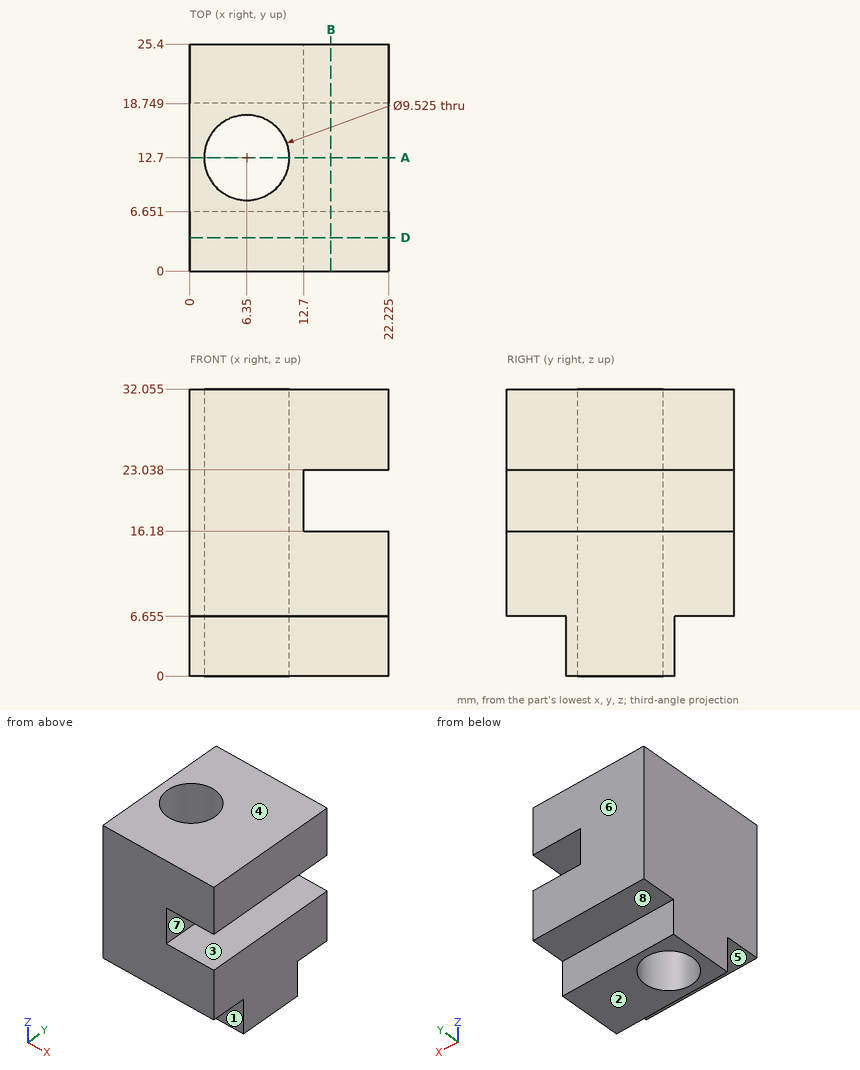
The figure shows three views and two pictorial views of one solid part (mm, origin at its lowest corner). Answer the questions. A direction names the side the tool comes from. Give positions to 0.01 mm unless a question says otherwise; leave off trailing zeros. Loops run counter-clockwise (first coordinate to the right, second up) from the corner with the lowest first, then second, coordinate; pieces in that order, holes last. Notation, with made-up numbers: (7, 34) -> (48, 34) arc R7 cw to (48, 47) -> close; hole circle Ø5 at (5.25, 51.5). An arc over 180 degrees is marked (long way). Put each result on its own line as item: value. Start each with the question number.
Item 1: Find the intervals of material crossed by L1, parallel to X at y = 12.7, z = 7 (1 decimal); L2, parallel to Z at x = 14.5, y = 13.75 (1 decimal); L3, parallel to Z at x = 19.5, y = 5.5 (1 decimal), in increasing order. Write a range as [from, to].
Item 2: Each of these flat-tipped pins is pushed along its axis until it touches: P1, Ø5.5, axis at x = 15, z = 2, coming from the +Y side; P2, Ø10, axis at y = 20, z = 13.5, coming from the -X side; P3, Ø3.5, axis at x = 10, y = 21, coming from the -Z side (3 decimals); P4, Ø2, axis at x = 5.5, z = 2, coming from the -Y side. Where does it stop, or does it pass through?
Item 3: Which of the six approach directions +Z, -Z, +X, -X, +Y, -Y give full straight-line access (tool end or side, diameter ignored) to the marked faces 5, 6, 7 and 8?
Item 4: The part is cut by section B-B (x = 15.75). Give the vertices of the cut face in (y, z) (1 decimal).
Item 5: The mould has two halves that part along Z. Classify the marked faces 1, 2, 3 and 4: released by +Z, released by -Z, zero draft, split by the parting line, or undercut.
Item 6: The part is cut by section D-D (y = 3.75). Give the vertices of the cut face in (x, z) (1 decimal).
Item 7: The part is cut by section A-A (y = 12.7). Give the vertices of the cut face in (x, z) (1 decimal), then the cut area to 3 significant figures.
Answers below:
1. L1: [0, 1.6], [11.1, 22.2]
1. L2: [0, 16.2], [23, 32.1]
1. L3: [6.7, 16.2], [23, 32.1]
2. P1: y = 18.75
2. P2: x = 0
2. P3: z = 6.655
2. P4: y = 6.65
3. face 5: -Z, +X, -X, -Y
3. face 6: +Z, -Z, +X, -X, +Y
3. face 7: +X, +Y, -Y
3. face 8: -Z, +X, -X, +Y
4. outline: (0, 6.7) -> (6.7, 6.7) -> (6.7, 0) -> (18.7, 0) -> (18.7, 6.7) -> (25.4, 6.7) -> (25.4, 16.2) -> (0, 16.2) -> close; (0, 23) -> (25.4, 23) -> (25.4, 32.1) -> (0, 32.1) -> close
5. face 1: zero draft
5. face 2: released by -Z
5. face 3: undercut
5. face 4: released by +Z
6. outline: (0, 6.7) -> (22.2, 6.7) -> (22.2, 16.2) -> (12.7, 16.2) -> (12.7, 23) -> (22.2, 23) -> (22.2, 32.1) -> (0, 32.1) -> close
7. outline: (0, 0) -> (1.6, 0) -> (1.6, 32.1) -> (0, 32.1) -> close; (11.1, 0) -> (22.2, 0) -> (22.2, 16.2) -> (12.7, 16.2) -> (12.7, 23) -> (22.2, 23) -> (22.2, 32.1) -> (11.1, 32.1) -> close
7. area: 342 mm2
